Design review of the part built by this model. Coordinates are the model's own, in mm. A direction names the side the tool comes from. Give positions to 0.01 mm unless a question says otherwise; leave off trailing zeros. Loops run counter-clockwise (first coordinate to the right, second up) from the corner with the lowest first, then second, coordinate; pieces in that order, holes last. Notation, with made-up numbers: (68, 20.25) -> (93, 20.25) arc R20 cw to (93, 24.25) -> close; hole circle Ø7 at (79, -17). An arc over 180 degrees is marked (long way). Answer in a Markdown table with one row per item. Add a question column.
(1) Consider section C-C on y = -0.5. Write out the cut boundary in (x, z), then the cut area to 3 significant figures.
(2) Consider section B-B on z = 0. Write out the cut boundary in (x, y).
(3) For line 1 (Y direction, x = 2.25, z = -2.5); line 2 (Z direction, x = 0, y = 23); line 3 (X direction, y = 20, z = 0), list the stretches that pass through material, from the lowest coordinate up.
(4) For pin 1 (1.5 mm diameter, centred on x = -2, y = 2, fed in from -Z); pin 2 (2 mm diameter, centred on x = 0.5, y = 10.5, fed in from +Z); pin 3 (1 mm diameter, centred on y = 18.5, z = -0.5, fed in from +X), all flat-tipped, find the tip position at first contact; note any pin that passes through.
(5) Consider section D-D on x = -3. Write out the cut boundary in (y, z), then the cut area to 3 significant figures.
(6) Consider section A-A on x = 0. Write out the cut boundary in (y, z), then the cut area to 3 significant figures.
(7) For faces 1 (the flat face through (0, 11, 1.5)), 2 (the flat face through (3, 29.8, 0)), 3 (the cylindrical face through (-3.612, 30.293, -0.802)), list the 3-axis set-ups (+Z, -Z, +X, -X, +Y, -Y) from which the entire face can be reached by the end or side of a thin tool; tool diameter is ignored.
from build123d import *

# Parameters (mm, degrees)
EXTRUDE_1_DEPTH = 27.8
SKETCH_2_R      = 2.5
EXTRUDE_2_DEPTH = 2
SKETCH_3_R      = 3.7
EXTRUDE_3_DEPTH = 1
EXTRUDE_START   = 2
EXTRUDE_4_DEPTH = 2
EXTRUDE_START_2 = 3
EXTRUDE_5_DEPTH = 3


with BuildPart() as part:
    # 草图1 → 凸台-拉伸1 (new body)
    with BuildSketch(Plane(origin=(0, 0, 0), x_dir=(1, 0, 0), z_dir=(0, 1, 0))):
        with BuildLine():
            Line((-2, -1.5), (2, -1.5))
            ThreePointArc((2, -1.5), (0, 2.5), (-2, -1.5))
        make_face()
    extrude(amount=EXTRUDE_1_DEPTH)

    # 草图2 → 凸台-拉伸2 (add)
    with BuildSketch(Plane(origin=(0, 27.8, 0), x_dir=(1, 0, 0), z_dir=(0, 1, 0))):
        with Locations(Location((0, 0, 0), (0, 0, 216.869897646))):
            Circle(SKETCH_2_R)
    extrude(amount=EXTRUDE_2_DEPTH)

    # 草图3 → 凸台-拉伸3 (add)
    with BuildSketch(Plane(origin=(0, 29.8, 0), x_dir=(1, 0, 0), z_dir=(0, 1, 0))):
        with Locations(Location((0, 0, 0), (0, 0, 270))):
            Circle(SKETCH_3_R)
    extrude(amount=EXTRUDE_3_DEPTH)

    # 草图4 → 凸台-拉伸4 (add)
    with BuildSketch(Plane.XZ.offset(EXTRUDE_START)):
        with BuildLine():
            Line((-2, 1.5), (2, 1.5))
            ThreePointArc((2, 1.5), (0, -2.5), (-2, 1.5))
        make_face()
    extrude(amount=-EXTRUDE_4_DEPTH)

    # 草图5 → 凸台-拉伸5 (add)
    with BuildSketch(Plane.XZ.offset(2).offset(EXTRUDE_START_2)):
        with BuildLine():
            Line((-2, 1.5), (2, 1.5))
            ThreePointArc((2, 1.5), (0, -2.5), (-2, 1.5))
        make_face()
    extrude(amount=-EXTRUDE_5_DEPTH)


solid = part.part
Values follow:
| question | item | result |
|---|---|---|
| 1 | outline | (-2, 1.5) arc R2.5 ccw (long way) to (2, 1.5) -> close |
| 1 | area | 16.8 mm2 |
| 2 | outline | (-3.7, 29.8) -> (-2.5, 29.8) -> (-2.5, -5) -> (2.5, -5) -> (2.5, 29.8) -> (3.7, 29.8) -> (3.7, 30.8) -> (-3.7, 30.8) -> close |
| 3 | line 1 | 29.8 to 30.8 |
| 3 | line 2 | -2.5 to 1.5 |
| 3 | line 3 | -2.5 to 2.5 |
| 4 | pin 1 | z = -2.17 |
| 4 | pin 2 | z = 1.5 |
| 4 | pin 3 | x = 2.5 |
| 5 | outline | (29.8, -2.17) -> (30.8, -2.17) -> (30.8, 2.17) -> (29.8, 2.17) -> close |
| 5 | area | 4.33 mm2 |
| 6 | outline | (-5, -2.5) -> (29.8, -2.5) -> (29.8, -3.7) -> (30.8, -3.7) -> (30.8, 3.7) -> (29.8, 3.7) -> (29.8, 2.5) -> (27.8, 2.5) -> (27.8, 1.5) -> (-5, 1.5) -> close |
| 6 | area | 149 mm2 |
| 7 | face 1 | +Z, +X, -X, -Y |
| 7 | face 2 | -Y |
| 7 | face 3 | +Y, -Y |
